Answer from the drawing. Dimensions are ordinates in mm from the lowest x, y and z of the part. Give positions to 0.01 mm unless a question says otherwise; leave off trailing zeros. Write each loop counter-clockwise with the first axis right and the second up, starting at its lowest first coordinate (ties: lowest second). Pieces come first, ordered by that corner, then holes. Notation, with made-up numbers: (-10, -2) -> (27, -2) arc R24 cw to (27, 33) -> close; hole circle Ø7 at (-10.75, 66.25). An arc over 180 degrees is marked (long way). Use a Markdown table: item, result. Add a question column.
Q1. Section D-D, the plane x = 145.5 is taken. Give the vertices of the cut face in (y, z).
Q2. Section B-B, the plane x = 5 is taken. Give the vertices of the cut face in (y, z).
Q3. Consider line 1 (X direction, y = 0.4, z = 5); line 2 (X direction, y = 74.5, z = 3.75); line 3 (Z direction, x = 179, y = 1.45). Determine where each line is inside the solid, lowest interval first.
Q4. Section C-C, the plane y = 71 is taken. Give the vertices of the cut face in (x, z).
Q5. Section A-A, the plane z = 5 is taken. Give the vertices of the cut face in (x, y), plus the area to 3 significant figures.
Q6. Each of these flat-tipped pins is pushed along its axis until it touches: pin 1 Ø5 at (y, z) = (42, 3) entering from -X; pin 2 Ø5 at (y, z) = (37, 7.5) entering from +X; pin 3 Ø1 at (x, z) = (19.5, 5) entering from -Y; pin 4 Ø4.5 at (x, z) = (5, 5) entering from +Y. Where does it stop, or does it pass through?
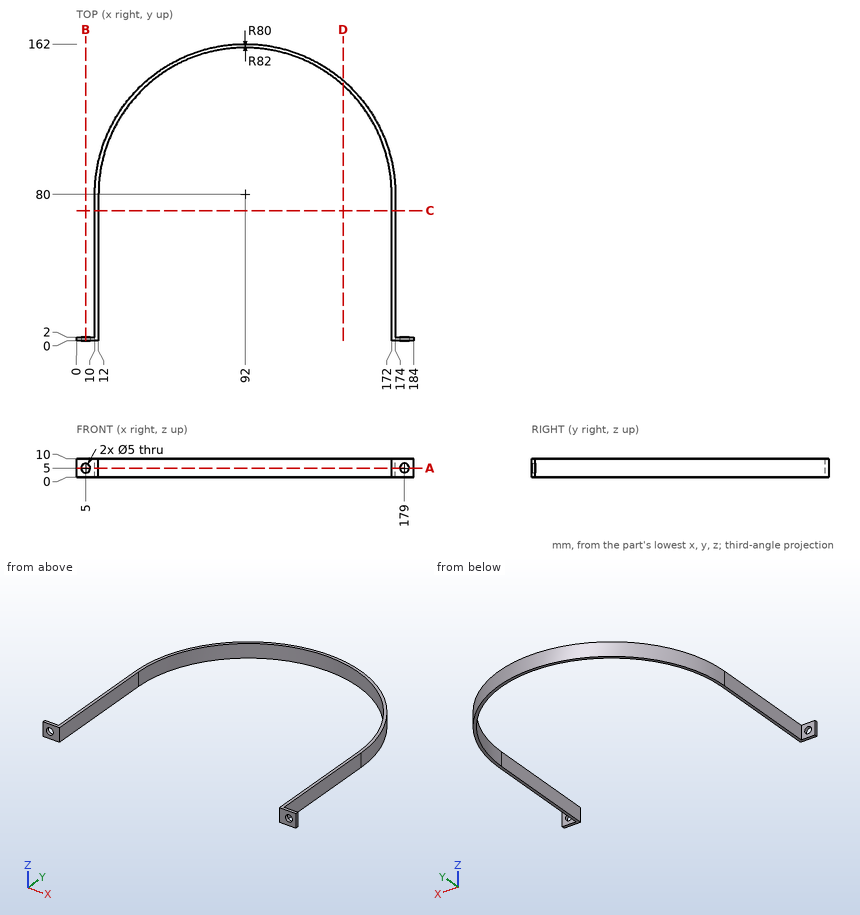
Result set:
| question | item | result |
|---|---|---|
| 1 | outline | (139.48, 0) -> (142.14, 0) -> (142.14, 10) -> (139.48, 10) -> close |
| 2 | outline | (0, 0) -> (2, 0) -> (2, 2.5) -> (0, 2.5) -> close; (0, 7.5) -> (2, 7.5) -> (2, 10) -> (0, 10) -> close |
| 3 | line 1 | x = 0 to 2.5, 7.5 to 12, 172 to 176.5, 181.5 to 184 |
| 3 | line 2 | x = 10 to 12, 172 to 174 |
| 3 | line 3 | z = 0 to 2.5, 7.5 to 10 |
| 4 | outline | (10, 0) -> (12, 0) -> (12, 10) -> (10, 10) -> close; (172, 0) -> (174, 0) -> (174, 10) -> (172, 10) -> close |
| 5 | outline | (0, 0) -> (2.5, 0) -> (2.5, 2) -> (0, 2) -> close; (7.5, 0) -> (12, 0) -> (12, 80) arc R80 cw to (172, 80) -> (172, 0) -> (176.5, 0) -> (176.5, 2) -> (174, 2) -> (174, 80) arc R82 ccw to (10, 80) -> (10, 2) -> (7.5, 2) -> close; (181.5, 0) -> (184, 0) -> (184, 2) -> (181.5, 2) -> close |
| 5 | area | 849 mm2 |
| 6 | pin 1 | stops at x = 10 |
| 6 | pin 2 | stops at x = 174 |
| 6 | pin 3 | stops at y = 112.73 |
| 6 | pin 4 | passes through |
